Part model, mm, in its own coordinate system. Face numbers are marked on the shaded views. A direction names the side the tool comes from. Coordinates: 2 decimals unless noted, no trailing zeros. Loops run counter-clockwise (first coordinate to the right, second up) from the corner with the lowest first, then second, coordinate; pieces in that order, holes last. Notation, with made-up numbers: (73, 83.5) - (115, 83.5) arc R15 ccw to (115, 111.5) - close; hole circle Ø11 at (41.25, 60.25). An arc over 180 degrees is marked (long way). Use a Markdown table: item, result. Add a question column.
1) Tool access for the marked faces 5 and 6: list every direction of +Z, -Z, +X, -X, +Y, -Y with a clear straight run to the whole face (end or side of a thin tool).
2) Pull direction X, two halves, no side cores. Call the marked faces 1, 2, 3 and 4: +X half, -X half, draft (parallel to the pull), parting line (faces both ways), or undercut.
3) Band-saw the part on C-C (x = 5). Give the number of separate pieces and of enclosed holes in the cut face, plus the area to 3 significant figures.
4) Drop flat-ended pins along their axis: P1, Ø1, axis at x = 18.5, z = 10, coming from the +Y side; P2, Ø8, axis at x = 5, y = -17, coming from the -Z side; P3, Ø8, axis at x = -0.5, z = 19.5, coming from the +Y side; P4, Ø11, axis at x = 6.47, z = 8.5, coming from the -Y side. Give the stop position or say it passes through.
5) Probe probe 1 along X at (y, z) = (-31.3, 8.5); probe 2 along X at (y, z) = (-16.5, 13.5); probe 3 along Y at (x, z) = (-2, 4). List the from-to ranges inside material, lowest first. Write a range as [from, to].
6) Band-saw the part on A-A (y = -30). Give the cut face in (x, z), plus the area to 3 significant figures.
7) Band-saw the part on B-B (z = 22.5). Give the cut face in (x, y).
from build123d import *

# Parameters (mm, degrees)
BOSS_EXTRUDE1_DEPTH = 28
CUT_EXTRUDE1_DEPTH  = 34.177233055
CUT_EXTRUDE2_DEPTH  = 17
SKETCH7_R           = 6.5
CUT_EXTRUDE3_DEPTH  = 29.0000001
SKETCH8_R           = 7
CUT_EXTRUDE4_DEPTH  = 10


with BuildPart() as part:
    # Sketch1 → Boss-Extrude1 (new body)
    with BuildSketch(Plane.XY):
        with BuildLine():
            Line((-10.121301077, -4.327557758), (-10.121301077, -33.827557937))
            Line((-10.121301077, -33.827557937), (23.055931978, -33.827557937))
            Line((23.055931978, -33.827557937), (23.055931978, -4.327557758))
            ThreePointArc((23.055931978, -4.327557758), (6.467315451, 12.261058769), (-10.121301077, -4.327557758))
        make_face()
    extrude(amount=BOSS_EXTRUDE1_DEPTH)

    # Sketch3 → Cut-Extrude1 (cut, through all)
    with BuildSketch(Plane(origin=(23.055931978, 0, 0), x_dir=(0, 0, -1), z_dir=(1, 0, 0))):
        with BuildLine():
            Line((0, -7.671360057), (0, -27.738941231))
            add(Edge.make_bspline(
                [(0, -27.738941231), (-8.213527787, -17.773605897), (-16, 12.261058769)],
                knots=[0, 0, 0, 1, 1, 1], degree=2))
            Line((-16, 12.261058769), (0, 12.261058769))
            Line((0, 12.261058769), (0, -7.671360057))
        make_face()
    extrude(amount=-CUT_EXTRUDE1_DEPTH, mode=Mode.SUBTRACT)

    # Sketch5 → Cut-Extrude2 (cut)
    with BuildSketch(Plane(origin=(0, 0, 0), x_dir=(-1, 0, 0), z_dir=(0, 0, -1))):
        with BuildLine():
            Line((-20.055931978, -28.827557937), (-20.055931978, -5.827557937))
            ThreePointArc((-20.055931978, -5.827557937), (-6.467315451, 7.76105859), (7.121301077, -5.827557937))
            Line((7.121301077, -5.827557937), (7.121301077, -28.827557937))
            Line((7.121301077, -28.827557937), (-20.055931978, -28.827557937))
        make_face()
    extrude(amount=-CUT_EXTRUDE2_DEPTH, mode=Mode.SUBTRACT)

    # Sketch7 → Cut-Extrude3 (cut, through all)
    with BuildSketch(Plane(origin=(0, 0, 0), x_dir=(-1, 0, 0), z_dir=(0, 0, -1))):
        with Locations((-6.068714161, -5.827557937)):
            Circle(SKETCH7_R)
    extrude(amount=-CUT_EXTRUDE3_DEPTH, mode=Mode.SUBTRACT)

    # Sketch8 → Cut-Extrude4 (cut)
    with BuildSketch(Plane(origin=(0, -28.827557937, 0), x_dir=(1, 0, 0), z_dir=(0, 1, 0))):
        with Locations((6.467315451, -8.5)):
            Circle(SKETCH8_R)
    extrude(amount=-CUT_EXTRUDE4_DEPTH, mode=Mode.SUBTRACT)


solid = part.part
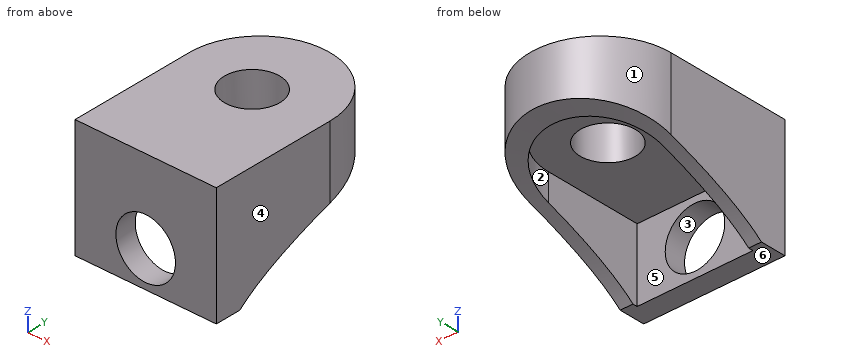
Answer block:
| question | item | result |
|---|---|---|
| 1 | face 5 | -Z |
| 1 | face 6 | -Z, +X, -X, +Y, -Y |
| 2 | face 1 | parting line |
| 2 | face 2 | undercut |
| 2 | face 3 | undercut |
| 2 | face 4 | +X half |
| 3 | separate pieces | 3 |
| 3 | enclosed holes | 0 |
| 3 | area | 389 mm2 |
| 4 | P1 | y = -28.83 |
| 4 | P2 | z = 17 |
| 4 | P3 | y = 11.99 |
| 4 | P4 | through |
| 5 | probe 1 | [-10.12, -0.53], [13.47, 23.06] |
| 5 | probe 2 | [-10.12, -7.12], [20.06, 23.06] |
| 5 | probe 3 | [-33.83, -28.83] |
| 6 | outline | (-10.12, 0) - (23.06, 0) - (23.06, 28) - (-10.12, 28) - close; hole circle Ø14 at (6.47, 8.5) |
| 6 | area | 775 mm2 |
| 7 | outline | (-10.12, -33.83) - (23.06, -33.83) - (23.06, -4.33) arc R16.59 ccw to (-10.12, -4.33) - close; hole circle Ø13 at (6.07, -5.83) |
